from build123d import *

# Parameters (mm, degrees)
ESQUISSE1_R        = 1.55
ESQUISSE1_W        = 5
ESQUISSE1_H        = 7
ESQUISSE1_W_2      = 2.5
ESQUISSE1_H_2      = 16
ESQUISSE1_W_3      = 6.6
ESQUISSE1_H_3      = 1.65
BOSS_EXTRU_1_DEPTH = 3


with BuildPart() as part:
    # Esquisse1 → Boss.-Extru.1 (new body)
    with BuildSketch(Plane.XY):
        with BuildLine():
            Line((26.6, 27.5), (-36, 27.5))
            ThreePointArc((-36, 27.5), (-38.828427125, 26.328427125), (-40, 23.5))
            Line((-40, 23.5), (-40, -23.5))
            ThreePointArc((-40, -23.5), (-38.828427125, -26.328427125), (-36, -27.5))
            Line((-36, -27.5), (26.6, -27.5))
            Line((26.6, -27.5), (26.6, -23.5))
            Line((26.6, -23.5), (31.6, -23.5))
            Line((31.6, -23.5), (31.6, -27.5))
            Line((31.6, -27.5), (36, -27.5))
            ThreePointArc((36, -27.5), (38.828427125, -26.328427125), (40, -23.5))
            Line((40, -23.5), (40, 23.5))
            ThreePointArc((40, 23.5), (38.828427125, 26.328427125), (36, 27.5))
            Line((36, 27.5), (31.6, 27.5))
            Line((31.6, 27.5), (31.6, 23.5))
            Line((31.6, 23.5), (26.6, 23.5))
            Line((26.6, 23.5), (26.6, 27.5))
        make_face()
        with Locations((-36, -23.5)):
            Circle(ESQUISSE1_R, mode=Mode.SUBTRACT)
        with Locations((-36, 23.5)):
            Circle(ESQUISSE1_R, mode=Mode.SUBTRACT)
        with Locations((36, 23.5)):
            Circle(ESQUISSE1_R, mode=Mode.SUBTRACT)
        with Locations((36, -23.5)):
            Circle(ESQUISSE1_R, mode=Mode.SUBTRACT)
        with Locations((29.1, -7)):
            Rectangle(ESQUISSE1_W, ESQUISSE1_H, mode=Mode.SUBTRACT)
        with Locations((-0.4, 10)):
            Rectangle(ESQUISSE1_W_2, ESQUISSE1_H_2, mode=Mode.SUBTRACT)
        with Locations((-17.5, -14.675)):
            Rectangle(ESQUISSE1_W_3, ESQUISSE1_H_3, mode=Mode.SUBTRACT)
        with Locations((2.85, -17)):
            Rectangle(ESQUISSE1_W_2, ESQUISSE1_H, mode=Mode.SUBTRACT)
    extrude(amount=BOSS_EXTRU_1_DEPTH)


solid = part.part
The listing builds one solid part. Answer for the finished solid, in the listing's coordinates (mm). A direction names the side the tool comes from. Coordinates: 2 decimals unless noted, no trailing zeros. Write each loop counter-clockwise with the first axis right and the second up, starting at its lowest first coordinate (ties: lowest second). Pieces come first, ordered by that corner, then holes. Notation, with made-up numbers: (60.25, 37.25) - (102.25, 37.25) arc R23 ccw to (102.25, 54.25) - close; hole circle Ø4 at (17, 56.25). An arc over 180 degrees is marked (long way). Return JSON: item names as keys, results as strings.
1. The part is cut by section A-A on y = 9. Determine the outline of the cut face in (x, z).
Final values:
{"outline": "(-40, 0) - (-1.65, 0) - (-1.65, 3) - (-40, 3) - close; (0.85, 0) - (40, 0) - (40, 3) - (0.85, 3) - close"}
2. For a pull along Y with two mould halves and no side action, classify faces 1 (the face through (-1, 0, 0)), 2 (the face through (36.83, -22.19, 1.48)), 3 (the face through (38.859, 26.297, 1.479)) as +Y half, -Y half, draft (parallel to the pull), parting line (faces both ways), or undercut.
Final values:
{"face 1": "draft", "face 2": "undercut", "face 3": "+Y half"}
3. Consider line 1 along Y through (x, z) = (-36, 1); line 2 along X through (y, z) = (-24, 1.6); line 3 along X through (y, z) = (6, 0.25). Determine where each line is inside the solid, lowest interval first.
Final values:
{"line 1": "-27.5 to -25.05, -21.95 to 21.95, 25.05 to 27.5", "line 2": "-39.97 to -37.47, -34.53 to 26.6, 31.6 to 34.53, 37.47 to 39.97", "line 3": "-40 to -1.65, 0.85 to 40"}
4. Each of these flat-tipped pins is pushed along its axis until it touches: pin 1 Ø0.9 at (y, z) = (-24.5, 2) entering from +X; pin 2 Ø1 at (x, z) = (31, 1) entering from +Y; pin 3 Ø3 at (x, y) = (29, 6) entering from -Z; pin 4 Ø1.5 at (y, z) = (26, 1.5) entering from -X. Where does it stop, or does it pass through?
Final values:
{"pin 1": "x = 39.96", "pin 2": "y = 23.5", "pin 3": "z = 0", "pin 4": "x = -39.6"}
5. Which of the six approach directions +Z, -Z, +X, -X, +Y, -Y give full straight-line access (tool end or side, diameter ignored) to faces 4 (the face through (29, 23.5, 1)), 5 (the face through (-40, 0, 1)), 6 (the face through (0, 2, 1)), 7 (the face through (29, -23.5, 1)), 8 (the face through (-1, 0, 3))?
Final values:
{"face 4": "+Z, -Z, +Y", "face 5": "+Z, -Z, -X, +Y, -Y", "face 6": "+Z, -Z", "face 7": "+Z, -Z, -Y", "face 8": "+Z, +X, -X, +Y, -Y"}
6. The part is cut by section B-B on x = -19. Determine the outline of the cut face in (y, z).
Final values:
{"outline": "(-27.5, 0) - (-15.5, 0) - (-15.5, 3) - (-27.5, 3) - close; (-13.85, 0) - (27.5, 0) - (27.5, 3) - (-13.85, 3) - close"}
7. The part is cut by section C-C on z = 1.25. Count the separate pieces of the cut face and the enclosed holes in it, then the cut area to 3 significant figures.
Final values:
{"separate pieces": "1", "enclosed holes": "8", "area": "4,210 mm^2"}
